Geometry check sheet. Reference: the model listing, model coordinates, mm. A direction names the side the tool comes from. Coordinates: 2 decimals unless noted, no trailing zeros. Write each loop counter-clockwise with the first axis right and the second up, starting at its lowest first coordinate (ties: lowest second). Pieces come first, ordered by that corner, then holes. Notation, with made-up numbers: M 81,89 L 100,89 A12 cw 100,101 Z; hole C 46.5,-26 d8. An arc over 180 degrees is marked long. Answer as a JSON object with one key per item and string values. Group by question number.
```python
from build123d import *

# Parameters (mm, degrees)
SK_SHROUD_W             = 25.86
SK_SHROUD_H             = 8.3
SHROUD_DEPTH            = 9.9
SK_FLANGE_EARS_W        = 3.4
SK_FLANGE_EARS_H        = 5.6
FLANGE_EARS_DEPTH       = 6
SK_CAVITY_W             = 23.86
SK_CAVITY_H             = 7.2
CAVITY_DEPTH            = 7.6
SK_TERMINAL_BLOCK_W     = 23.65
SK_TERMINAL_BLOCK_H     = 11.75
TERMINAL_BLOCK_DEPTH    = 10.1
INSERT_HOLES_DEPTH      = 25.590016267
INSERT_HOLES_DEPTH_BACK = 25.590016267
SK_INSERT_HOLES_R       = 1.25
SK_CONTACT_PINS_W       = 1
SK_CONTACT_PINS_H       = 1
CONTACT_PINS_DEPTH      = 6
SK_WIRE_ENTRIES_W       = 2.6
SK_WIRE_ENTRIES_H       = 2.8
WIRE_ENTRIES_DEPTH      = 6
SK_CLAMP_SCREW_HOLES_R  = 1.3
CLAMP_SCREW_HOLES_DEPTH = 3


with BuildPart() as part:
    # SK Shroud → Shroud (new body)
    with BuildSketch(Plane.XY.offset(3)):
        with Locations((0, -0.6)):
            Rectangle(SK_SHROUD_W, SK_SHROUD_H)
    extrude(amount=-SHROUD_DEPTH)

    # SK Flange ears → Flange ears (add)
    with BuildSketch(Plane.XY.offset(3)):
        with Locations((14.63, 0)):
            Rectangle(SK_FLANGE_EARS_W, SK_FLANGE_EARS_H)
        with Locations((-14.63, 0)):
            Rectangle(SK_FLANGE_EARS_W, SK_FLANGE_EARS_H)
    extrude(amount=-FLANGE_EARS_DEPTH)

    # SK Cavity → Cavity (cut)
    with BuildSketch(Plane.XY.offset(3)):
        with Locations((0, -0.6)):
            Rectangle(SK_CAVITY_W, SK_CAVITY_H)
    extrude(amount=-CAVITY_DEPTH, mode=Mode.SUBTRACT)

    # SK Terminal block → Terminal block (add)
    with BuildSketch(Plane.XY.offset(-6.9)):
        with Locations((0, 1.125)):
            Rectangle(SK_TERMINAL_BLOCK_W, SK_TERMINAL_BLOCK_H)
    extrude(amount=-TERMINAL_BLOCK_DEPTH)

    # SK Insert holes → Insert holes (cut, two sides: drawn at the far end of the back side and taken through both)
    with BuildSketch(Plane.XY.offset(-INSERT_HOLES_DEPTH_BACK)):
        with Locations((-13.945, 0)):
            Circle(SK_INSERT_HOLES_R)
        with Locations((13.945, 0)):
            Circle(SK_INSERT_HOLES_R)
    extrude(amount=INSERT_HOLES_DEPTH + INSERT_HOLES_DEPTH_BACK, mode=Mode.SUBTRACT)

    # SK Contact pins → Contact pins (add)
    with BuildSketch(Plane.XY.offset(-4.6)):
        with Locations((-9.525, -0.6)):
            Rectangle(SK_CONTACT_PINS_W, SK_CONTACT_PINS_H)
        with Locations((-5.715, -0.6)):
            Rectangle(SK_CONTACT_PINS_W, SK_CONTACT_PINS_H)
        with Locations((-1.905, -0.6)):
            Rectangle(SK_CONTACT_PINS_W, SK_CONTACT_PINS_H)
        with Locations((1.905, -0.6)):
            Rectangle(SK_CONTACT_PINS_W, SK_CONTACT_PINS_H)
        with Locations((5.715, -0.6)):
            Rectangle(SK_CONTACT_PINS_W, SK_CONTACT_PINS_H)
        with Locations((9.525, -0.6)):
            Rectangle(SK_CONTACT_PINS_W, SK_CONTACT_PINS_H)
    extrude(amount=CONTACT_PINS_DEPTH)

    # SK Wire entries → Wire entries (cut)
    with BuildSketch(Plane.XY.offset(-17)):
        with Locations((-9.525, -2)):
            Rectangle(SK_WIRE_ENTRIES_W, SK_WIRE_ENTRIES_H)
        with Locations((-5.715, -2)):
            Rectangle(SK_WIRE_ENTRIES_W, SK_WIRE_ENTRIES_H)
        with Locations((-1.905, -2)):
            Rectangle(SK_WIRE_ENTRIES_W, SK_WIRE_ENTRIES_H)
        with Locations((1.905, -2)):
            Rectangle(SK_WIRE_ENTRIES_W, SK_WIRE_ENTRIES_H)
        with Locations((5.715, -2)):
            Rectangle(SK_WIRE_ENTRIES_W, SK_WIRE_ENTRIES_H)
        with Locations((9.525, -2)):
            Rectangle(SK_WIRE_ENTRIES_W, SK_WIRE_ENTRIES_H)
    extrude(amount=WIRE_ENTRIES_DEPTH, mode=Mode.SUBTRACT)

    # SK Clamp screw holes → Clamp screw holes (cut)
    with BuildSketch(Plane(origin=(0, 7, 0), x_dir=(1, 0, 0), z_dir=(0, 1, 0))):
        with Locations(Location((-9.525, 12, 0), (0, 0, 270))):
            Circle(SK_CLAMP_SCREW_HOLES_R)
        with Locations(Location((-5.715, 12, 0), (0, 0, 270))):
            Circle(SK_CLAMP_SCREW_HOLES_R)
        with Locations(Location((-1.905, 12, 0), (0, 0, 270))):
            Circle(SK_CLAMP_SCREW_HOLES_R)
        with Locations(Location((1.905, 12, 0), (0, 0, 270))):
            Circle(SK_CLAMP_SCREW_HOLES_R)
        with Locations(Location((5.715, 12, 0), (0, 0, 270))):
            Circle(SK_CLAMP_SCREW_HOLES_R)
        with Locations(Location((9.525, 12, 0), (0, 0, 270))):
            Circle(SK_CLAMP_SCREW_HOLES_R)
    extrude(amount=-CLAMP_SCREW_HOLES_DEPTH, mode=Mode.SUBTRACT)


solid = part.part
```
1) Section check B-B (x = 11.5). Record the cut outline in (y, z).
2) Draft check along X on faces 4 (the flat face through (-2, -0.6, -14)), 5 (the flat face through (2, -1.1, -2)). Enter one of: +X half, -X half, draft (parallel to the pull), parting line (faces both ways), or undercut.
3) Section check D-D (x = -14). Record the cut outline in (y, z), then the cut area to 3 significant figures.
4) Set-up check for faces 1 (the flat face through (6, 4, -12)), 2 (the flat face through (8.225, -2, -14)), 3 (the flat face through (1.9, -0.6, 1.4)): record each of +Z, -Z, +X, -X, +Y, -Y from which the full face is reachable in a straight line by a thin tool's end or side.
5) Go/stop test with flat-tipped pins: pin 1 Ø1.3 at (x, z) = (9.5, -11.5) entering from +Y; pin 2 Ø4 at (x, z) = (-5.5, -2) entering from +Y; pin 3 Ø3 at (y, z) = (-1, -7) entering from +X. Record where each tip stops, or that it passes through.
6) Section check A-A (z = 2). Record the cut outline in (x, y) (3 decimals).
7) Section check C-C (z = -5). Record the cut outline in (x, y) (3 decimals), then the cut area to 3 significant figures.
8) Material ranges on probe 1 along Y at (x, z) = (-3.5, -1.75); probe 2 along Y at (x, z) = (-10, -14.5); probe 3 along Y at (x, z) = (-5.5, -4.5), recorded low to high. Write a range as [from, to].
Entries:
{
 "1": {"outline": "M -4.75,-17 L 7,-17 L 7,-6.9 L 3.55,-6.9 L 3.55,3 L 3,3 L 3,-4.6 L -4.2,-4.6 L -4.2,3 L -4.75,3 Z"},
 "2": {"face 4": "undercut", "face 5": "undercut"},
 "3": {"outline": "M -2.8,-3 L -1.25,-3 L -1.25,3 L -2.8,3 Z; M 1.25,-3 L 2.8,-3 L 2.8,3 L 1.25,3 Z", "area": "18.6 mm^2"},
 "4": {"face 1": "+Y", "face 2": "-Z", "face 3": "+Z"},
 "5": {"pin 1": "y = 4", "pin 2": "y = 3.55", "pin 3": "x = 12.93"},
 "6": {"outline": "M -16.33,-2.8 L -12.93,-2.8 L -12.93,-4.75 L 12.93,-4.75 L 12.93,-2.8 L 16.33,-2.8 L 16.33,2.8 L 12.93,2.8 L 12.93,3.55 L -12.93,3.55 L -12.93,2.8 L -16.33,2.8 Z; hole C -13.945,0 d2.5; hole M -11.93,-4.2 L 11.93,-4.2 L 11.93,3 L -11.93,3 Z; hole C 13.945,0 d2.5"},
 "7": {"outline": "M -12.93,-4.75 L 12.93,-4.75 L 12.93,-0.73 A1.25 cw 12.93,0.73 L 12.93,3.55 L -12.93,3.55 L -12.93,0.73 A1.25 cw -12.93,-0.73 Z", "area": "214 mm^2"},
 "8": {"probe 1": "[-4.75, -4.2], [3, 3.55]", "probe 2": "[-4.75, -3.4], [-0.6, 7]", "probe 3": "[-4.75, -4.2], [-1.1, -0.1], [3, 3.55]"}
}
